Source: CAD feature listing. Evaluate the final solid. Frame: model axes, mm. Give positions to 0.01 mm unless a question says otherwise; leave off trailing zeros. Order: outer loops, then holes, each group sorted by start corner. A loop starts at its lowest first (then second) coordinate and runs counter-clockwise, first axis right, second up.
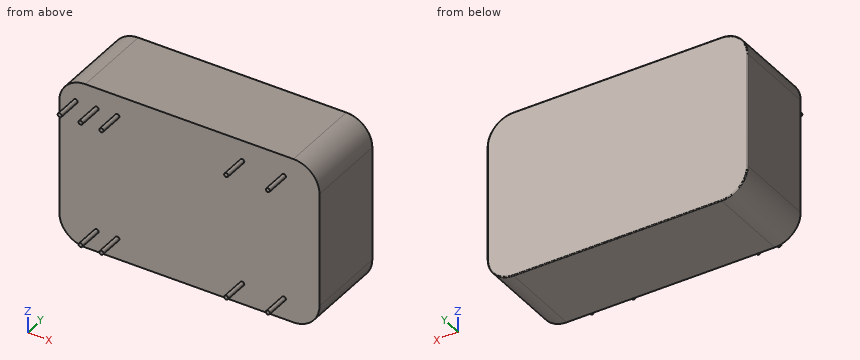
```python
from build123d import *

# Parameters (mm, degrees)
SKETCH1_W           = 31.75
SKETCH1_H           = 20.32
BOSS_EXTRUDE1_DEPTH = 10.16
SKETCH2_R           = 0.25
BOSS_EXTRUDE2_DEPTH = 3.05
FILLET1_R           = 3.18
FILLET2_R           = 0.1


with BuildPart() as part:
    # Sketch1 → Boss-Extrude1 (new body)
    with BuildSketch(Plane(origin=(0, 0, 0), x_dir=(1, 0, 0), z_dir=(0, 1, 0))):
        Rectangle(SKETCH1_W, SKETCH1_H)
    extrude(amount=BOSS_EXTRUDE1_DEPTH)

    # Sketch2 → Boss-Extrude2 (add)
    with BuildSketch(Plane.XZ):
        with Locations((-13.875, 7.62)):
            Circle(SKETCH2_R)
        with Locations((-11.335, 7.62)):
            Circle(SKETCH2_R)
        with Locations((-8.795, 7.62)):
            Circle(SKETCH2_R)
        with Locations((6.445, 7.62)):
            Circle(SKETCH2_R)
        with Locations((11.525, 7.62)):
            Circle(SKETCH2_R)
        with Locations((11.525, -7.62)):
            Circle(SKETCH2_R)
        with Locations((6.445, -7.62)):
            Circle(SKETCH2_R)
        with Locations((-8.795, -7.62)):
            Circle(SKETCH2_R)
        with Locations((-11.335, -7.62)):
            Circle(SKETCH2_R)
    extrude(amount=BOSS_EXTRUDE2_DEPTH)

    # Fillet1
    fillet1_edges = [part.edges().sort_by_distance(p)[0] for p in [
        (-15.875, 5.08, -10.16),
        (15.875, 5.08, -10.16),
        (15.875, 5.08, 10.16),
        (-15.875, 5.08, 10.16),
    ]]
    fillet(fillet1_edges, radius=FILLET1_R)

    # Fillet2
    fillet2_edges = [part.edges().sort_by_distance(p)[0] for p in [
        (0, 10.16, -10.16),
        (15.875, 10.16, 0),
        (-15.875, 10.16, 0),
        (0, 10.16, 10.16),
        (-14.943599564, 10.16, 9.228599564),
        (-14.943599564, 10.16, -9.228599564),
        (14.943599564, 10.16, 9.228599564),
        (14.943599564, 10.16, -9.228599564),
    ]]
    fillet(fillet2_edges, radius=FILLET2_R)


solid = part.part
```
1) Section query C-C, the plane x = -7.5. Return the cut outline in (y, z), and give its area (3 significant figures).
Report:
outline: (0, -10.16) - (10.06, -10.16) arc R0.1 ccw to (10.16, -10.06) - (10.16, 10.06) arc R0.1 ccw to (10.06, 10.16) - (0, 10.16) - close
area: 206 mm2
2) Section query A-A, the plane y = -0.5. Count the separate pieces of the cut face and the enclosed holes in it, and give its area (3 significant figures).
Report:
separate pieces: 9
enclosed holes: 0
area: 1.77 mm2
3) Pin query (flat end, axial travel): pin 1 (4 mm diameter, centred on x = 4.5, y = -0.5, fed in from -Z); pin 2 (1 mm diameter, centred on x = -8.5, z = 2.5, fed in from -Y). Return the tip coordinate at first contact, or that it passes through.
Report:
pin 1: stops at z = -10.16
pin 2: stops at y = 0
4) Section query B-B, the plane z = -0.75. Return the cut outline in (x, y) (3 decimals).
Report:
outline: (-15.875, 0) - (15.875, 0) - (15.875, 10.06) arc R0.1 ccw to (15.775, 10.16) - (-15.775, 10.16) arc R0.1 ccw to (-15.875, 10.06) - close
5) Material intervals for L1, parallel to Y at x = 1.5, z = 7.75; L2, parallel to X at y = 7.75, z = -9, sorted ascending.
Report:
L1: y = 0 to 10.16
L2: x = -15.15 to 15.15
